from build123d import *

# Parameters (mm, degrees)
BOSS_EXTRUDE1_DEPTH = 450
SKETCH2_R           = 50
BOSS_EXTRUDE2_DEPTH = 125
SKETCH3_R           = 50
BOSS_EXTRUDE3_DEPTH = 125
SKETCH4_R           = 50
CUT_EXTRUDE1_DEPTH  = 25
SKETCH5_W           = 100
SKETCH5_H           = 100
CUT_EXTRUDE2_DEPTH  = 25


with BuildPart() as part:
    # Sketch1 → Boss-Extrude1 (new body)
    with BuildSketch(Plane.XY):
        Polygon((-275, 500), (-275, 375), (275, 375), (275, 500), (500, 500), (500, -500), (275, -500), (275, -375), (-275, -375), (-275, -500), (-500, -500), (-500, 500), align=None)
    extrude(amount=BOSS_EXTRUDE1_DEPTH)

    # Sketch2 → Boss-Extrude2 (add)
    with BuildSketch(Plane.XZ.offset(375)):
        with Locations((0, 190)):
            Circle(SKETCH2_R)
    extrude(amount=BOSS_EXTRUDE2_DEPTH)

    # Sketch3 → Boss-Extrude3 (add)
    with BuildSketch(Plane(origin=(0, 375, 0), x_dir=(1, 0, 0), z_dir=(0, 1, 0))):
        with Locations((0, -190)):
            Circle(SKETCH3_R)
    extrude(amount=BOSS_EXTRUDE3_DEPTH)

    # Sketch4 → Cut-Extrude1 (cut)
    with BuildSketch(Plane.XY.offset(450)):
        Circle(SKETCH4_R)
    extrude(amount=-CUT_EXTRUDE1_DEPTH, mode=Mode.SUBTRACT)

    # Sketch5 → Cut-Extrude2 (cut)
    with BuildSketch(Plane(origin=(0, 0, 0), x_dir=(-1, 0, 0), z_dir=(0, 0, -1))):
        with Locations((350, 0)):
            Rectangle(SKETCH5_W, SKETCH5_H)
        with Locations((-350, 0)):
            Rectangle(SKETCH5_W, SKETCH5_H)
    extrude(amount=-CUT_EXTRUDE2_DEPTH, mode=Mode.SUBTRACT)


solid = part.part
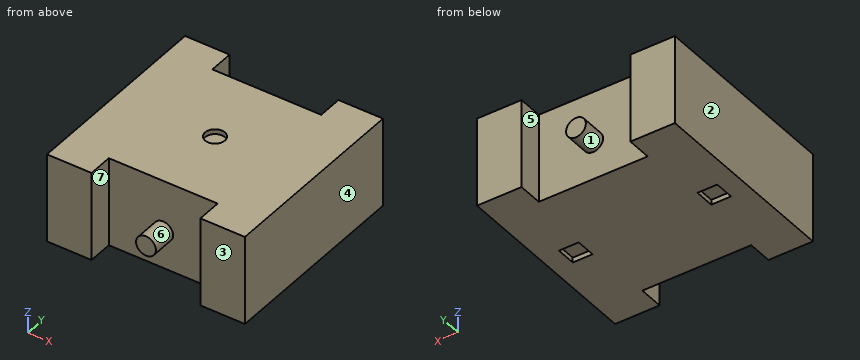
For this review, take the finished solid that the model builds, in its own axes (mm). Face numbers are marked on the shaded views. A direction names the side the tool comes from. Round coordinates to 2 decimals unless told otherwise and drop trailing zeros. Loops run counter-clockwise (first coordinate to the right, second up) from the corner with the lowest first, then second, coordinate; pieces in that order, holes last. Notation, with made-up numbers: (84, 39) - (141, 39) arc R18 cw to (141, 53) - close; hole circle Ø7 at (-20, 60.5). An arc over 180 degrees is marked (long way). Use one line per item in the form item = value.
1) Wall thickness on probe 1 along X at (y, z) = (48, 20); probe 2 along Y at (x, z) = (0, 431.5); probe 3 along X at (y, z) = (397, 359): over which ranges is each line inside the solid? List them lowest first.
Solutions:
probe_1 = -500 to -400, -300 to 300, 400 to 500
probe_2 = -375 to -50, 50 to 375
probe_3 = -500 to -275, 275 to 500
2) We need section B-B on x = 0. Write out the cut boundary in (y, z).
Solutions:
outline = (-500, 140) - (-375, 140) - (-375, 0) - (375, 0) - (375, 140) - (500, 140) - (500, 240) - (375, 240) - (375, 450) - (50, 450) - (50, 425) - (-50, 425) - (-50, 450) - (-375, 450) - (-375, 240) - (-500, 240) - close
3) We need section C-C on y = 0. Write out the cut boundary in (x, z), then the cut area to 4 significant figures.
Solutions:
outline = (-500, 0) - (-400, 0) - (-400, 25) - (-300, 25) - (-300, 0) - (300, 0) - (300, 25) - (400, 25) - (400, 0) - (500, 0) - (500, 450) - (50, 450) - (50, 425) - (-50, 425) - (-50, 450) - (-500, 450) - close
area = 442,500 mm2
4) We need section D-D on z = 266. Write out the cut boundary in (x, y).
Solutions:
outline = (-500, -500) - (-275, -500) - (-275, -375) - (275, -375) - (275, -500) - (500, -500) - (500, 500) - (275, 500) - (275, 375) - (-275, 375) - (-275, 500) - (-500, 500) - close
5) Clearance check with a flat-ended pin moving along its axis: P1, Ø4, axis at x = 144.5, z = 49.5, coming from the +Y side. State where the tip first meets the part, or that it passes through.
Solutions:
P1 = 375
6) Mouldability with a two-part tool opening along X and no side actions: class the marked faces 1, 2, 3 and 4 as pulls with the +X half, pulls with the -X half, needs draft (parallel to the pull), parting line crosses it, or undercut.
Solutions:
face_1 = undercut
face_2 = pulls with the -X half
face_3 = needs draft
face_4 = pulls with the +X half
7) Tool access review of the marked faces 5, 6 and 7: name each direction out of +Z, -Z, +X, -X, +Y, -Y from which nothing blocks a thin tool from reaching the whole face with its end or side.
Solutions:
face_5 = +Z, -Z, +Y
face_6 = -Y
face_7 = +Z, -Z, -Y
8) We need section A-A on y = -425. Write out the cut boundary in (x, z), then the cut area to 3 significant figures.
Solutions:
outline = (-500, 0) - (-275, 0) - (-275, 450) - (-500, 450) - close; circle Ø100 at (0, 190); (275, 0) - (500, 0) - (500, 450) - (275, 450) - close
area = 210,000 mm2
